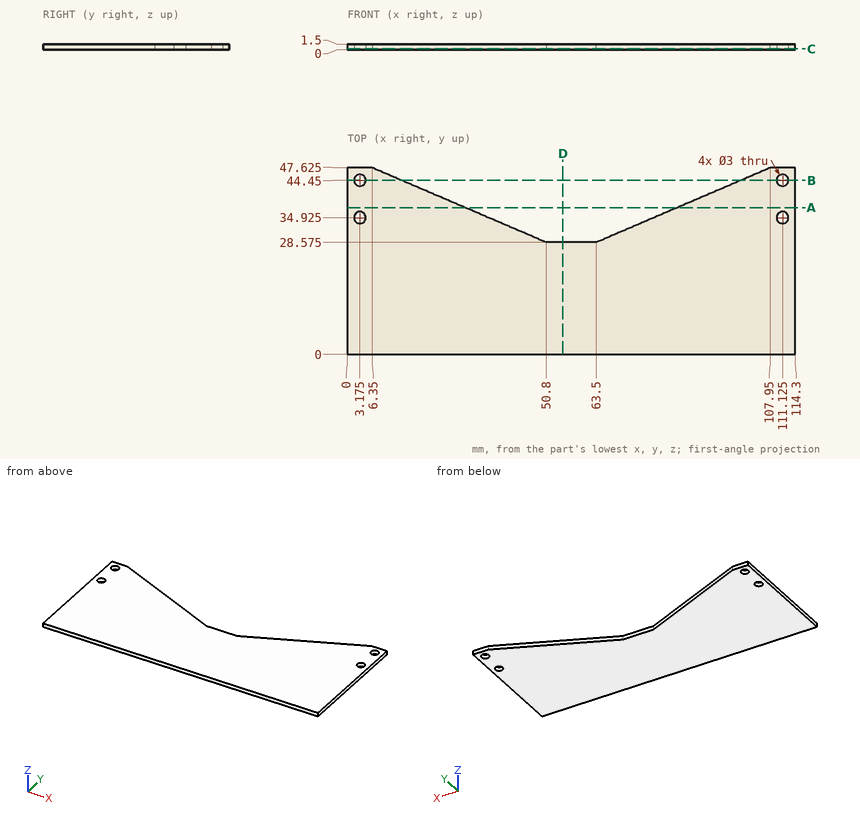
The figure shows three views and two pictorial views of one solid part (mm, origin at its lowest corner). Answer the questions. Coordinates: 2 decimals unless noted, no trailing zeros. Write each loop counter-clockwise with the first axis right and the second up, starting at its lowest first coordinate (ties: lowest second). Pieces come first, ordered by that corner, then holes.
1. The part is cut by section D-D, the plane x = 55. Write down the section's boundary in (y, z) (3 decimals).
Results list:
outline: (0, 0) - (28.575, 0) - (28.575, 1.5) - (0, 1.5) - close
2. The part is cut by section B-B, the plane y = 44.45. Write down the section's boundary in (x, z) (3 decimals).
Results list:
outline: (0, 0) - (1.675, 0) - (1.675, 1.5) - (0, 1.5) - close; (4.675, 0) - (13.758, 0) - (13.758, 1.5) - (4.675, 1.5) - close; (100.542, 0) - (109.625, 0) - (109.625, 1.5) - (100.542, 1.5) - close; (112.625, 0) - (114.3, 0) - (114.3, 1.5) - (112.625, 1.5) - close
3. Consider line 1 along Y through (x, z) = (56.5, 1.35) (3 decimals); line 2 along X through (y, z) = (39, 0.65) (3 decimals); line 3 along Y through (x, z) = (33, 1.05). Determine where each line is inside the solid, lowest interval first.
Results list:
line 1: y = 0 to 28.575
line 2: x = 0 to 26.475, 87.825 to 114.3
line 3: y = 0 to 36.2
4. The part is cut by section C-C, the plane z = 0.25. Write down the section's boundary in (x, y) (3 decimals).
Results list:
outline: (0, 0) - (114.3, 0) - (114.3, 47.625) - (107.95, 47.625) - (63.5, 28.575) - (50.8, 28.575) - (6.35, 47.625) - (0, 47.625) - close; hole circle Ø3 at (3.175, 34.925); hole circle Ø3 at (3.175, 44.45); hole circle Ø3 at (111.125, 34.925); hole circle Ø3 at (111.125, 44.45)
5. The part is cut by section A-A, the plane y = 37.5. Write down the section's boundary in (x, z) (3 decimals).
Results list:
outline: (0, 0) - (29.975, 0) - (29.975, 1.5) - (0, 1.5) - close; (84.325, 0) - (114.3, 0) - (114.3, 1.5) - (84.325, 1.5) - close
